Check sheet for the drawn part. Datum: minimum x, y, z corner. Units: mm. Round coordinates to 2 decimals unless told otherwise and drop trailing zeros. Write each loop counter-clockwise with the first axis right and the second up, starting at its lowest first coordinate (ties: lowest second). Pieces come first, ordered by that corner, then holes. Notation, with made-up numbers: (1, -40) - (57, -40) arc R4 cw to (57, -34) - close; hole circle Ø5 at (21, -33.75). An arc over 180 degrees is marked (long way). Answer as a JSON object with one key per item and string values. Group by question number.
Item 1: Gauge pin test, flat ends, axial feed: P1, Ø1.5, axis at y = 23, z = 3, coming from the +X side; P2, Ø1.5, axis at x = 5.5, z = 1.5, coming from the +Y side; P3, Ø1.5, axis at x = 144.5, z = 2.5, coming from the -Y side. Record the tip position at first contact, or that the pin passes through.
Item 2: Sectioned sample at B-B on y = 14.5. Record the boundary of the cut face in (x, z).
Item 3: Sectioned sample at C-C on z = 2.8. Record the boundary of the cut face in (x, y).
Item 4: Sectioned sample at D-D on x = 141.5. Record the boundary of the cut face in (y, z).
Item 5: Thickness scan on line 1 (Y direction, x = 75, z = 3.4); line 2 (X direction, y = 19.5, z = 1); line 3 (X direction, y = 9, z = 0.8). Record the ranges inside material, lowest first.
Item 6: Sectioned sample at A-A on x = 75. Record the boundary of the cut face in (y, z), plus the area to 3 significant figures.
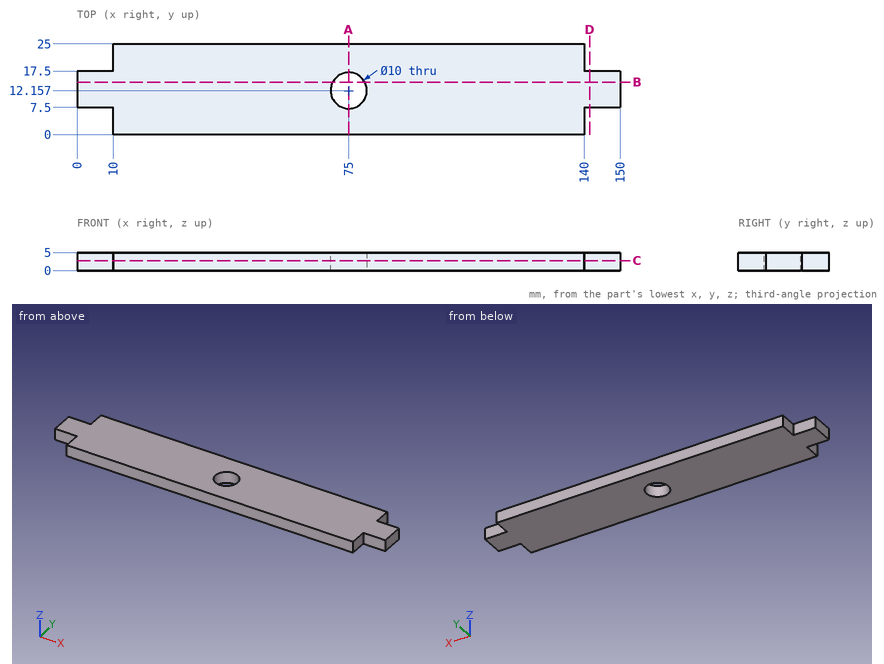
Completed:
{
 "1": {"P1": "x = 140", "P2": "y = 17.5", "P3": "y = 7.5"},
 "2": {"outline": "(0, 0) - (70.58, 0) - (70.58, 5) - (0, 5) - close; (79.42, 0) - (150, 0) - (150, 5) - (79.42, 5) - close"},
 "3": {"outline": "(0, 7.5) - (10, 7.5) - (10, 0) - (140, 0) - (140, 7.5) - (150, 7.5) - (150, 17.5) - (140, 17.5) - (140, 25) - (10, 25) - (10, 17.5) - (0, 17.5) - close; hole circle Ø10 at (75, 12.16)"},
 "4": {"outline": "(7.5, 0) - (17.5, 0) - (17.5, 5) - (7.5, 5) - close"},
 "5": {"line 1": "0 to 7.16, 17.16 to 25", "line 2": "10 to 140", "line 3": "0 to 71.12, 78.88 to 150"},
 "6": {"outline": "(0, 0) - (7.16, 0) - (7.16, 5) - (0, 5) - close; (17.16, 0) - (25, 0) - (25, 5) - (17.16, 5) - close", "area": "75.0 mm²"}
}
